Read the model definition and answer for the solid it produces. Units are mm, in the model's axes. Face numbers are marked on the shaded views. A direction names the side the tool comes from. Round coordinates to 2 decimals unless told otherwise and drop trailing zeros. Write each loop counter-clockwise with the first axis right and the second up, starting at its lowest first coordinate (ties: lowest second). Pieces come first, ordered by that corner, then holes. Notation, with made-up numbers: (80.5, 69) -> (130.5, 69) arc R23 cw to (130.5, 81) -> close; hole circle Ø5 at (87.25, 32). An arc over 180 degrees is marked (long way). Return JSON: item names as keys, results as strings.
from build123d import *

# Parameters (mm, degrees)
SKETCH_3_R          = 10.85
EXTRUDE_1_DEPTH     = 5.5
SKETCH_4_R          = 14
EXTRUDE_2_DEPTH     = 4
SKETCH_5_R          = 4
SKETCH_5_R_2        = 1.6
CUT_EXTRUDE_1_DEPTH = 50


with BuildPart() as part:
    # 草图3 → 凸台-拉伸1 (new body)
    with BuildSketch(Plane(origin=(0, 0, 0), x_dir=(1, 0, 0), z_dir=(0, 1, 0))):
        with Locations(Location((0, 0, 0), (0, 0, 270))):
            Circle(SKETCH_3_R)
    extrude(amount=EXTRUDE_1_DEPTH)

    # 草图4 → 凸台-拉伸2 (add)
    with BuildSketch(Plane(origin=(0, 5.5, 0), x_dir=(1, 0, 0), z_dir=(0, 1, 0))):
        with Locations(Location((0, 0, 0), (0, 0, 270))):
            Circle(SKETCH_4_R)
    extrude(amount=EXTRUDE_2_DEPTH)

    # 草图5 → 切除-拉伸1 (cut)
    with BuildSketch(Plane(origin=(0, 9.5, 0), x_dir=(1, 0, 0), z_dir=(0, 1, 0))):
        with Locations(Location((0, 0, 0), (0, 0, 270))):
            Circle(SKETCH_5_R)
        with Locations(Location((0, 7, 0), (0, 0, 270))):
            Circle(SKETCH_5_R_2)
        with Locations(Location((7, 0, 0), (0, 0, 270))):
            Circle(SKETCH_5_R_2)
        with Locations(Location((0, -7, 0), (0, 0, 270))):
            Circle(SKETCH_5_R_2)
        with Locations(Location((-7, 0, 0), (0, 0, 270))):
            Circle(SKETCH_5_R_2)
    extrude(amount=-CUT_EXTRUDE_1_DEPTH, mode=Mode.SUBTRACT)


solid = part.part
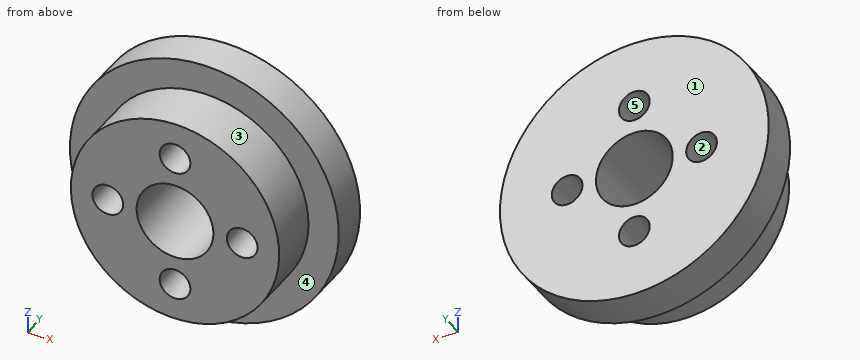
Item 1: Section B-B (z = 0) is taken. Give the vertices of the cut face in (x, y).
Worked answers:
{"outline": "(-14, 5.5) -> (-10.85, 5.5) -> (-10.85, 0) -> (-8.6, 0) -> (-8.6, 9.5) -> (-14, 9.5) -> close; (-5.4, 0) -> (-4, 0) -> (-4, 9.5) -> (-5.4, 9.5) -> close; (4, 0) -> (5.4, 0) -> (5.4, 9.5) -> (4, 9.5) -> close; (8.6, 0) -> (10.85, 0) -> (10.85, 5.5) -> (14, 5.5) -> (14, 9.5) -> (8.6, 9.5) -> close"}
Item 2: Section D-D (z = 7) is taken. Give the vertices of the cut face in (x, y).
Worked answers:
{"outline": "(-12.12, 5.5) -> (-8.29, 5.5) -> (-8.29, 0) -> (-1.6, 0) -> (-1.6, 9.5) -> (-12.12, 9.5) -> close; (1.6, 0) -> (8.29, 0) -> (8.29, 5.5) -> (12.12, 5.5) -> (12.12, 9.5) -> (1.6, 9.5) -> close"}
Item 3: A tool of negligible diameter and unlimited length cuts with its end or side. For the marked faces 4 and 5, from which of +Z, -Z, +X, -X, +Y, -Y can it reach the whole face along a straight path? Write none if from no direction.
Worked answers:
{"face 4": "-Y", "face 5": "+Y, -Y"}
Item 4: For a pull along Z with two mould halves and no side action, classify the marked faces 1, 2 and 3 as released by +Z, released by -Z, zero draft, split by the parting line, or undercut.
Worked answers:
{"face 1": "zero draft", "face 2": "undercut", "face 3": "split by the parting line"}
Item 5: Flat-ended cylindrical pins translate along their axes: pin 1 (2 mm diameter, centred on y = 3.5, z = -9.5, fed in from -X); pin 2 (3 mm diameter, centred on y = 3, z = -8.5, fed in from -X); pin 3 (3 mm diameter, centred on y = 7, z = 11, fed in from +X). Find the tip coordinate at first contact, or state that the pin passes through.
Worked answers:
{"pin 1": "stops at x = -6.74", "pin 2": "stops at x = -8.29", "pin 3": "stops at x = 10.28"}
Item 6: Straight lines are drawn through the part: L1, parallel to X at y = 6, z = 0; L2, parallel to Y at x = -9.25, z = 9.75; L3, parallel to X at y = 3.5, z = 1. For each, find the intervals that lie inside material, in ascending order. Write a range as [from, to].
Worked answers:
{"L1": "x = [-14, -8.6], [-5.4, -4], [4, 5.4], [8.6, 14]", "L2": "y = [5.5, 9.5]", "L3": "x = [-10.8, -8.25], [-5.75, -3.87], [3.87, 5.75], [8.25, 10.8]"}
Item 7: Section C-C (y = 6) is taken. Give the vertices of the cut face in (x, z).
Worked answers:
{"outline": "circle Ø28 at (0, 0); hole circle Ø3.2 at (-7, 0); hole circle Ø8 at (0, 0); hole circle Ø3.2 at (0, -7); hole circle Ø3.2 at (0, 7); hole circle Ø3.2 at (7, 0)"}
Item 8: Section A-A (x = 0) is taken. Give the vertices of the cut face in (y, z).
Worked answers:
{"outline": "(0, -10.85) -> (5.5, -10.85) -> (5.5, -14) -> (9.5, -14) -> (9.5, -8.6) -> (0, -8.6) -> close; (0, -5.4) -> (9.5, -5.4) -> (9.5, -4) -> (0, -4) -> close; (0, 4) -> (9.5, 4) -> (9.5, 5.4) -> (0, 5.4) -> close; (0, 8.6) -> (9.5, 8.6) -> (9.5, 14) -> (5.5, 14) -> (5.5, 10.85) -> (0, 10.85) -> close"}
